The model under review builds one solid part; all positions refer to its coordinate system, in mm. Face numbers are marked on the shaded views. A direction names the side the tool comes from. Round coordinates to 2 decimals unless told otherwise and drop trailing zeros. Order: outer loops, then holes, each group sorted by start corner. A loop starts at its lowest first (then second) coordinate and runs counter-clockwise, first axis right, second up. Notation, with made-up numbers: M 50,75.5 L 81,75.5 A31 ccw 81,100.5 Z; hole C -18,-39 d11. An arc over 180 degrees is marked long. Use a Markdown table: item, result. Add a question column.
1. The part is to be moulded in two halves that separate along Y. For the marked faces 4, 5 and 6, say which applies: +Y half, -Y half, draft (parallel to the pull), parting line (faces both ways), or undercut.
2. Consider section B-B on z = 113.5. State the section outline as (x, y) points, then the cut area to 3 significant figures.
3. Consider section C-C on z = 287.5. State the section outline as (x, y) points.
4. Consider section A-A on z = 489. State the section outline as (x, y) points.
5. Insertion check: P1, Ø12, axis at x = -595.5, z = 349, coming from the -Y side; P2, Ø5, axis at y = 112, z = 190.5, coming from the +X side; P3, Ø6, axis at y = -357, z = 139.5, coming from the +X side. Each pin has a flat end and moves straight along its axis. Give the tip position at first contact, or say it passes through.
6. For the marked faces 1, 2 and 3, list the 3-axis set-ups (+Z, -Z, +X, -X, +Y, -Y) from which the entire face can be reached by the end or side of a thin tool; tool diameter is ignored.
7. To check wall thickness, follow probe 1 along Y at (x, z) = (0, 177); probe 2 along Z at (x, y) = (-348, -246); probe 3 along Y at (x, z) = (161.5, 612). State the ranges of each line that lie inside material, in increasing order.
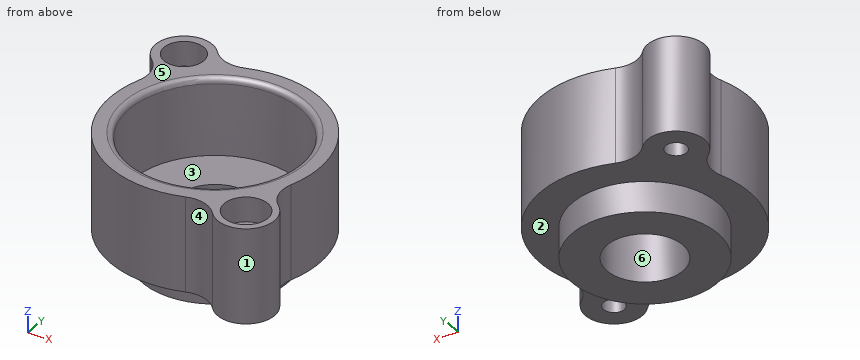
from build123d import *

# Parameters (mm, degrees)
BOSS_EXTRU_1_DEPTH      = 635
ESQUISSE2_R             = 486.41
BOSS_EXTRU_2_DEPTH      = 203.2
ESQUISSE3_R             = 572.77
ENL_V_MAT_EXTRU_1_DEPTH = 508
ENL_V_MAT_EXTRU_1_TAPER = 1.432096184
ESQUISSE4_R             = 254
ENL_V_MAT_EXTRU_2_DEPTH = 331.2
PER_AGE1_D              = 139.7
PER_AGE1_DEPTH          = 838.2
PER_AGE1_CBORE_D        = 292.1
PER_AGE1_CBORE_DEPTH    = 165.1
PER_AGE2_D              = 139.7
PER_AGE2_DEPTH          = 838.2
PER_AGE2_CBORE_D        = 266.7
PER_AGE2_CBORE_DEPTH    = 165.1
CONG_1_R                = 38.1


with BuildPart() as part:
    # Esquisse1 → Boss.-Extru.1 (new body)
    with BuildSketch(Plane.XY.offset(838.2)):
        with BuildLine():
            ThreePointArc((-229.773752251, 659.625858177), (-350.063866609, 655.471932336), (-451.601786597, 720.101782381))
            ThreePointArc((-451.601786597, 720.101782381), (-731.603841816, 731.603841816), (-720.101782381, 451.601786597))
            ThreePointArc((-720.101782381, 451.601786597), (-655.471932336, 350.063866609), (-659.625858178, 229.773752251))
            ThreePointArc((-659.625858178, 229.773752251), (-493.914086659, -493.914086659), (229.773752251, -659.625858178))
            ThreePointArc((229.773752251, -659.625858178), (350.063866609, -655.471932336), (451.601786596, -720.101782381))
            ThreePointArc((451.601786596, -720.101782381), (731.603841816, -731.603841816), (720.101782381, -451.601786596))
            ThreePointArc((720.101782381, -451.601786596), (655.471932336, -350.063866609), (659.625858178, -229.773752251))
            ThreePointArc((659.625858178, -229.773752251), (493.914086659, 493.914086659), (-229.773752251, 659.625858177))
        make_face()
    extrude(amount=-BOSS_EXTRU_1_DEPTH)

    # Esquisse2 → Boss.-Extru.2 (add)
    with BuildSketch(Plane(origin=(0, 0, 203.2), x_dir=(-1, 0, 0), z_dir=(0, 0, -1))):
        Circle(ESQUISSE2_R)
    extrude(amount=BOSS_EXTRU_2_DEPTH)

    # Esquisse3 → Enlèv. mat.-Extru.1 (cut)
    with BuildSketch(Plane.XY.offset(838.2)):
        Circle(ESQUISSE3_R)
    extrude(amount=-ENL_V_MAT_EXTRU_1_DEPTH, taper=ENL_V_MAT_EXTRU_1_TAPER, mode=Mode.SUBTRACT)

    # Esquisse4 → Enlèv. mat.-Extru.2 (cut, through all)
    with BuildSketch(Plane.XY.offset(330.2)):
        Circle(ESQUISSE4_R)
    extrude(amount=-ENL_V_MAT_EXTRU_2_DEPTH, mode=Mode.SUBTRACT)

    # Perçage1
    with Locations(Plane.XY.offset(838.2)):
        with Locations((596.9, -596.9)):
            CounterBoreHole(PER_AGE1_D / 2, PER_AGE1_CBORE_D / 2, PER_AGE1_CBORE_DEPTH, depth=PER_AGE1_DEPTH)

    # Perçage2
    with Locations(Plane.XY.offset(838.2)):
        with Locations((-596.9, 596.9)):
            CounterBoreHole(PER_AGE2_D / 2, PER_AGE2_CBORE_D / 2, PER_AGE2_CBORE_DEPTH, depth=PER_AGE2_DEPTH)

    # Congé1
    cong_1_edges = [part.edges().sort_by_distance(p)[0] for p in [
        (-572.77, 0, 838.2),
    ]]
    fillet(cong_1_edges, radius=CONG_1_R)


solid = part.part
Answer block:
| question | item | result |
|---|---|---|
| 1 | face 4 | -Y half |
| 1 | face 5 | draft |
| 1 | face 6 | undercut |
| 2 | outline | C 0,0 d972.82; hole C 0,0 d508 |
| 2 | area | 541,000 mm^2 |
| 3 | outline | M -720.1,451.6 A203.2 cw -659.63,229.77 A698.5 ccw 229.77,-659.63 A203.2 cw 451.6,-720.1 A190.5 ccw long 720.1,-451.6 A203.2 cw 659.63,-229.77 A698.5 ccw -229.77,659.63 A203.2 cw -451.6,720.1 A190.5 ccw long Z; hole C -596.9,596.9 d139.7; hole C 0,0 d508; hole C 596.9,-596.9 d139.7 |
| 4 | outline | M -720.1,451.6 A203.2 cw -659.63,229.77 A698.5 ccw 229.77,-659.63 A203.2 cw 451.6,-720.1 A190.5 ccw long 720.1,-451.6 A203.2 cw 659.63,-229.77 A698.5 ccw -229.77,659.63 A203.2 cw -451.6,720.1 A190.5 ccw long Z; hole C -596.9,596.9 d139.7; hole C 0,0 d1128.08; hole C 596.9,-596.9 d139.7 |
| 5 | P1 | y = -374.69 |
| 5 | P2 | x = 473.92 |
| 5 | P3 | x = 333.58 |
| 6 | face 1 | +Z, -Z |
| 6 | face 2 | -Z |
| 6 | face 3 | +Z |
| 7 | probe 1 | -486.41 to -254, 254 to 486.41 |
| 7 | probe 2 | 0 to 330.2 |
| 7 | probe 3 | -679.57 to -543.63, 543.63 to 679.57 |
